from build123d import *

# Parameters (mm, degrees)
F0_R      = 9.525
F1_DEPTH  = 12.7
F1_FACE_R = 9.525
F2_DEPTH  = 25.4


with BuildPart() as f1:
    # F0 (on Front) → F1 (new body)
    with BuildSketch(Plane.XZ):
        with BuildLine():
            Line((-79.602955, 0), (-21.997045, 0))
            ThreePointArc((-21.997045, 0), (-10.998523, 6.35), (-10.998523, 19.05))
            Line((-10.998523, 19.05), (-39.801477, 68.938181))
            ThreePointArc((-39.801477, 68.938181), (-50.8, 75.288181), (-61.798523, 68.938181))
            Line((-61.798523, 68.938181), (-90.601477, 19.05))
            ThreePointArc((-90.601477, 19.05), (-90.601477, 6.35), (-79.602955, 0))
        make_face()
        with Locations((-74.103693, 15.875)):
            Circle(F0_R, mode=Mode.SUBTRACT)
        with Locations((-27.496307, 15.875)):
            Circle(F0_R, mode=Mode.SUBTRACT)
        with Locations((-50.8, 29.329394)):
            Circle(F0_R, mode=Mode.SUBTRACT)
        with Locations((-50.8, 56.238181)):
            Circle(F0_R, mode=Mode.SUBTRACT)
    extrude(amount=F1_DEPTH)

    # F1_face (on face) → F2 (join)
    with BuildSketch(Plane(origin=(-50.8, -12.7, 29.329394), x_dir=(1, 0, 0), z_dir=(0, -1, 0))):
        with BuildLine():
            Line((-28.802955, -29.329394), (28.802955, -29.329394))
            ThreePointArc((28.802955, -29.329394), (39.801477, -22.979394), (39.801477, -10.279394))
            Line((39.801477, -10.279394), (10.998523, 39.608787))
            ThreePointArc((10.998523, 39.608787), (0, 45.958787), (-10.998523, 39.608787))
            Line((-10.998523, 39.608787), (-39.801477, -10.279394))
            ThreePointArc((-39.801477, -10.279394), (-39.801477, -22.979394), (-28.802955, -29.329394))
        make_face()
        with Locations((-23.303693, -13.454394)):
            Circle(F1_FACE_R, mode=Mode.SUBTRACT)
        with Locations((23.303693, -13.454394)):
            Circle(F1_FACE_R, mode=Mode.SUBTRACT)
        Circle(F1_FACE_R, mode=Mode.SUBTRACT)
        with Locations((0, 26.908787)):
            Circle(F1_FACE_R, mode=Mode.SUBTRACT)
    extrude(amount=F2_DEPTH)


solid = f1.part
Could you check a few things on this model? Use its own coordinates, in mm. Give positions to 0.01 mm unless a question says otherwise; leave off trailing zeros. Order: outer loops, then holes, each group sorted by start corner. A loop starts at its lowest first (then second) coordinate and runs counter-clockwise, first axis right, second up. Notation, with made-up numbers: (-31, 66.25) - (-21, 66.25) arc R20 ccw to (-21, 103.25) - close; hole circle Ø11 at (83.25, -36). An arc over 180 degrees is marked (long way). One line per item, written item: value. Start each with the question number.
1. Imagine slicing it at D-D on y = -20. List the corners of the cut face in (x, z) for me (3 decimals).
2. Thinking about a two-plate mould opening in Z: for faces 1 (the face through (-46.4, -18.78, 20.88)), 2 (the face through (-90.693, -18.783, 6.512)), 3 (the face through (-18.4, -18.8, 18.7)), 4 (the face through (-51, -19, 0)), which applies, +Z half, -Z half, draft (parallel to the pull), parting line (faces both ways), or undercut?
3. Imagine slicing it at B-B on z = 57.5. List the corners of the cut face in (x, y) for me, plus the area to 3 significant figures.
4. If I drill on probe 1 along X at (y, z) = (-22, 9); probe 2 along Z at (x, y) = (-56, -2.5); probe 3 along Z at (x, y) = (-57.5, -24), over which ranges is the centre line in solid material (lowest first)?
5. Imagine slicing it at C-C on x = -71. List the corners of the cut face in (y, z) for me.
6. Imagine slicing it at A-A on x = -50.8. List the corners of the cut face in (y, z) for me.
7. For P1, Ø1.5, axis at y = -10.5, z = 54.5, coming from the -X side; P2, Ø12, axis at y = -8.5, z = 30, coming from the -X side; P3, Ø6, axis at x = -61.5, y = -27.5, coming from the +Z side; P4, Ø17, axis at x = -50.8, z = 29.33, coming from the -Y side, each with a flat end and sliding along its axis, tell me the tip position at first contact or that it passes through.
Values:
1. outline: (-90.601, 19.05) arc R12.7 ccw to (-79.603, 0) - (-21.997, 0) arc R12.7 ccw to (-10.999, 19.05) - (-39.801, 68.938) arc R12.7 ccw to (-61.799, 68.938) - close; hole circle Ø19.05 at (-74.104, 15.875); hole circle Ø19.05 at (-50.8, 29.329); hole circle Ø19.05 at (-50.8, 56.238); hole circle Ø19.05 at (-27.496, 15.875)
2. face 1: undercut
2. face 2: parting line
2. face 3: undercut
2. face 4: -Z half
3. outline: (-68.4, -38.1) - (-60.24, -38.1) - (-60.24, 0) - (-68.4, 0) - close; (-41.36, -38.1) - (-33.2, -38.1) - (-33.2, 0) - (-41.36, 0) - close
3. area: 622 mm²
4. probe 1: -91.75 to -80.7, -67.51 to -34.09, -20.9 to -9.85
4. probe 2: 0 to 21.35, 37.31 to 48.26, 64.22 to 74.17
4. probe 3: 0 to 22.56, 36.1 to 49.47, 63.01 to 73.38
5. outline: (-38.1, 0) - (0, 0) - (0, 6.87) - (-38.1, 6.87) - close; (-38.1, 24.88) - (0, 24.88) - (0, 53) - (-38.1, 53) - close
6. outline: (-38.1, 0) - (0, 0) - (0, 19.8) - (-38.1, 19.8) - close; (-38.1, 38.85) - (0, 38.85) - (0, 46.71) - (-38.1, 46.71) - close; (-38.1, 65.76) - (0, 65.76) - (0, 75.29) - (-38.1, 75.29) - close
7. P1: x = -70.57
7. P2: x = -87.74
7. P3: z = 72.69
7. P4: through
